Read the model definition and answer for the solid it produces. Units are mm, in the model's axes. A direction names the side the tool comes from. Give positions to 0.01 mm unless a question says otherwise; leave off trailing zeros. Write each loop counter-clockwise with the first axis right and the second up, starting at its lowest first coordinate (ties: lowest second). Pieces come first, ordered by that corner, then holes. Notation, with made-up numbers: (-12.5, 13.25) - (2.5, 13.25) arc R17 cw to (2.5, 25.25) - close; hole circle Ø10 at (78, -17.5). An arc over 180 degrees is marked (long way). Answer as a JSON object with one key per item and string values. Group by question number.
```python
from build123d import *

# Parameters (mm, degrees)
SKETCH1_W                  = 58.6
SKETCH1_H                  = 20.38979341
BRACKETBASE_DEPTH          = 5
SKETCH2_W                  = 20.38979341
SKETCH2_H                  = 12
LEGMOUNTINGTAB_DEPTH       = 5
SKETCH3_R                  = 2.125
LEGMOUNTINGHOLES_DEPTH     = 5
SKETCH4_W                  = 20.38979341
SKETCH4_H                  = 7
ARDUINOMOUNTINGTAB_DEPTH   = 4.38979341
SKETCH5_R                  = 2.125
ARDUINOMOUNTINGHOLES_DEPTH = 5
FILLET1_R                  = 2
BOSS_EXTRUDE1_DEPTH        = 13.38979341
SKETCH7_R                  = 2.125
BOSS_EXTRUDE2_DEPTH        = 4.38979341
CUT_EXTRUDE1_DEPTH         = 69.695127089
CUT_EXTRUDE1_DEPTH_BACK    = 69.695127089
BOSS_EXTRUDE3_DEPTH        = 58.6


with BuildPart() as part:
    # Sketch1 → bracketBase (new body)
    with BuildSketch(Plane(origin=(0, 0, 0), x_dir=(1, 0, 0), z_dir=(0, 1, 0))):
        with Locations((29.3, 10.194896705)):
            Rectangle(SKETCH1_W, SKETCH1_H)
    extrude(amount=BRACKETBASE_DEPTH)

    # Sketch2 → legMountingTab (add)
    with BuildSketch(Plane.ZY):
        with Locations((-10.194896705, 6)):
            Rectangle(SKETCH2_W, SKETCH2_H)
    legmountingtab = extrude(amount=-LEGMOUNTINGTAB_DEPTH)

    # Sketch3 → legMountingHoles (cut)
    with BuildSketch(Plane(origin=(5, 0, 0), x_dir=(0, 0, -1), z_dir=(1, 0, 0))):
        with Locations((15.13979341, 8.75)):
            Circle(SKETCH3_R)
        with Locations((5.13979341, 8.75)):
            Circle(SKETCH3_R)
    legmountingholes = extrude(amount=-LEGMOUNTINGHOLES_DEPTH, mode=Mode.SUBTRACT)

    # legMountingHoles2: legMountingTab, legMountingHoles across plane
    add(legmountingtab.mirror(Plane.ZY.offset(-29.3)))
    add(legmountingholes.mirror(Plane.ZY.offset(-29.3)), mode=Mode.SUBTRACT)

    # Sketch4 → arduinoMountingTab (add)
    with BuildSketch(Plane.XY):
        with Locations((29.3, -3.5)):
            Rectangle(SKETCH4_W, SKETCH4_H)
    extrude(amount=-ARDUINOMOUNTINGTAB_DEPTH)

    # Sketch5 → arduinoMountingHoles (cut)
    with BuildSketch(Plane.XY):
        with Locations((34.397448352, -3.5)):
            Circle(SKETCH5_R)
        with Locations(Location((24.202551647, -3.5, 0), (0, 0, 180))):
            Circle(SKETCH5_R)
    extrude(amount=-ARDUINOMOUNTINGHOLES_DEPTH, mode=Mode.SUBTRACT)

    # Fillet1
    fillet1_edges = [part.edges().sort_by_distance(p)[0] for p in [
        (39.494896705, 0, -2.194896705),
        (39.494896705, -7, -2.194896705),
        (19.105103295, -7, -2.194896705),
        (19.105103295, 0, -2.194896705),
    ]]
    fillet(fillet1_edges, radius=FILLET1_R)

    # Sketch6 → Boss-Extrude1 (add)
    with BuildSketch(Plane(origin=(0, 0, -20.38979341), x_dir=(-1, 0, 0), z_dir=(0, 0, -1))):
        Polygon((-5, 5), (-53.6, 5), (-53.6, 12), (-58.6, 12), (-58.6, 0), (0, 0), (0, 12), (-5, 12), align=None)
    extrude(amount=BOSS_EXTRUDE1_DEPTH)

    # Sketch7 → Boss-Extrude2 (add)
    with BuildSketch(Plane(origin=(0, 0, -33.77958682), x_dir=(-1, 0, 0), z_dir=(0, 0, -1))):
        with BuildLine():
            Line((-37.494896705, -7), (-21.105103295, -7))
            ThreePointArc((-21.105103295, -7), (-19.690889733, -6.414213562), (-19.105103295, -5))
            Line((-19.105103295, -5), (-19.105103295, -2))
            ThreePointArc((-19.105103295, -2), (-18.519316857, -0.585786438), (-17.105103295, 0))
            Line((-17.105103295, 0), (-41.494896705, 0))
            ThreePointArc((-41.494896705, 0), (-40.080683143, -0.585786438), (-39.494896705, -2))
            Line((-39.494896705, -2), (-39.494896705, -5))
            ThreePointArc((-39.494896705, -5), (-38.909110267, -6.414213562), (-37.494896705, -7))
        make_face()
        with Locations(Location((-34.397448352, -3.5, 0), (0, 0, 180))):
            Circle(SKETCH7_R, mode=Mode.SUBTRACT)
        with Locations((-24.202551647, -3.5)):
            Circle(SKETCH7_R, mode=Mode.SUBTRACT)
    extrude(amount=-BOSS_EXTRUDE2_DEPTH)

    # Sketch8 → Cut-Extrude1 (cut, two sides: drawn at the far end of the back side and taken through both)
    with BuildSketch(Plane(origin=(58.6, 0, 0), x_dir=(0, 0, -1), z_dir=(1, 0, 0)).offset(-CUT_EXTRUDE1_DEPTH_BACK)):
        Polygon((20.38979341, 12), (33.77958682, 5), (33.77958682, 12), align=None)
    extrude(amount=CUT_EXTRUDE1_DEPTH + CUT_EXTRUDE1_DEPTH_BACK, mode=Mode.SUBTRACT)

    # Sketch9 → Boss-Extrude3 (add)
    with BuildSketch(Plane.ZY):
        Polygon((-20.38979341, 12), (-20.38979341, 5), (-33.77958682, 5), align=None)
    extrude(amount=-BOSS_EXTRUDE3_DEPTH)


solid = part.part
```
1) Find section A-A, the plane y = -3.5. Write down the section's boundary in (x, z), and give its area (3 significant figures).
2) Find section B-B, the plane z = -6.5. Write down the section's boundary in (x, y), and give its area (3 significant figures).
3) Find the intervals of material crossed by line 1 (X direction, y = 9.75, z = -1); line 2 (Y direction, x = 49, z = -16); line 3 (Y direction, x = 35, z = -4), in increasing order. Write a range as [from, to].
4) Flat-ended cylindrical pins translate along their axes: pin 1 Ø2 at (x, y) = (41, -4.5) entering from +Z; pin 2 Ø3.5 at (x, y) = (19, 8.5) entering from +Z; pin 3 Ø2.5 at (y, z) = (-3, -1.5) entering from +X; pin 4 Ø0.9 at (y, z) = (-3, -2.5) entering from -X. Find the tip coordinate at first contact, or state that the pin passes through.
5) For a pull along Y with two mould halves and no side action, classify faces 4 (the cylindrical face through (22.24, -4.31, -31.62)), 5 (the cylindrical face through (40.096, -0.57, -31.615)), 6 (the flat face through (53.6, 8, -10)) as released by +Y, released by -Y, zero draft, split by the parting line, or undercut.
6) Find section C-C, the plane y = 8.75. Write down the section's boundary in (x, z).
7) Which of the six approach directions +Z, -Z, +X, -X, +Y, -Y give full straight-line access (tool end or side, diameter ignored) to faces 1 (the flat face through (29, 5, -10)), 2 (the cylindrical face through (56.065, 6.865, -6.12)), 3 (the flat face through (39.495, -3, -32))?
Values follow:
{
 "1": {"outline": "(19.11, -33.78) - (22.08, -33.78) - (22.08, -29.39) - (19.11, -29.39) - close; (19.11, -4.39) - (22.08, -4.39) - (22.08, 0) - (19.11, 0) - close; (26.33, -33.78) - (32.27, -33.78) - (32.27, -29.39) - (26.33, -29.39) - close; (26.33, -4.39) - (32.27, -4.39) - (32.27, 0) - (26.33, 0) - close; (36.52, -33.78) - (39.49, -33.78) - (39.49, -29.39) - (36.52, -29.39) - close; (36.52, -4.39) - (39.49, -4.39) - (39.49, 0) - (36.52, 0) - close", "area": "104 mm2"},
 "2": {"outline": "(0, 0) - (58.6, 0) - (58.6, 7.12) - (53.6, 7.12) - (53.6, 5) - (5, 5) - (5, 7.12) - (0, 7.12) - close; (0, 10.38) - (5, 10.38) - (5, 12) - (0, 12) - close; (53.6, 10.38) - (58.6, 10.38) - (58.6, 12) - (53.6, 12) - close", "area": "330 mm2"},
 "3": {"line 1": "x = [0, 5], [53.6, 58.6]", "line 2": "y = [0, 5]", "line 3": "y = [-7, -5.54], [-1.46, 5]"},
 "4": {"pin 1": "passes through", "pin 2": "stops at z = -20.39", "pin 3": "stops at x = 39.51", "pin 4": "stops at x = 19.11"},
 "5": {"face 4": "undercut", "face 5": "released by -Y", "face 6": "zero draft"},
 "6": {"outline": "(0, -26.61) - (58.6, -26.61) - (58.6, -17.26) - (53.6, -17.26) - (53.6, -20.39) - (5, -20.39) - (5, -17.26) - (0, -17.26) - close; (0, -13.01) - (5, -13.01) - (5, -7.26) - (0, -7.26) - close; (0, -3.01) - (5, -3.01) - (5, 0) - (0, 0) - close; (53.6, -13.01) - (58.6, -13.01) - (58.6, -7.26) - (53.6, -7.26) - close; (53.6, -3.01) - (58.6, -3.01) - (58.6, 0) - (53.6, 0) - close"},
 "7": {"face 1": "+Z, +Y", "face 2": "+X, -X", "face 3": "+Z, -Z, +X, -Y"}
}
